Could you check a few things on this drawing? It's one solid part, dimensions in mm from its lowest x, y, z. A direction names the side the tool comes from. Round coordinates to 2 decimals unless told otherwise and drop trailing zeros. Loops run counter-clockwise (first coordinate to the right, second up) from the corner with the lowest first, then second, coordinate; pieces in that order, holes last. Notation, with made-up numbers: (50.5, -28.5) -> (99.5, -28.5) arc R21 cw to (99.5, 9.5) -> close; hole circle Ø6 at (-36, -6.5). An arc over 180 degrees is marked (long way). Use CSV: the item, a comma, the result in double quotes. Start each with the question number.
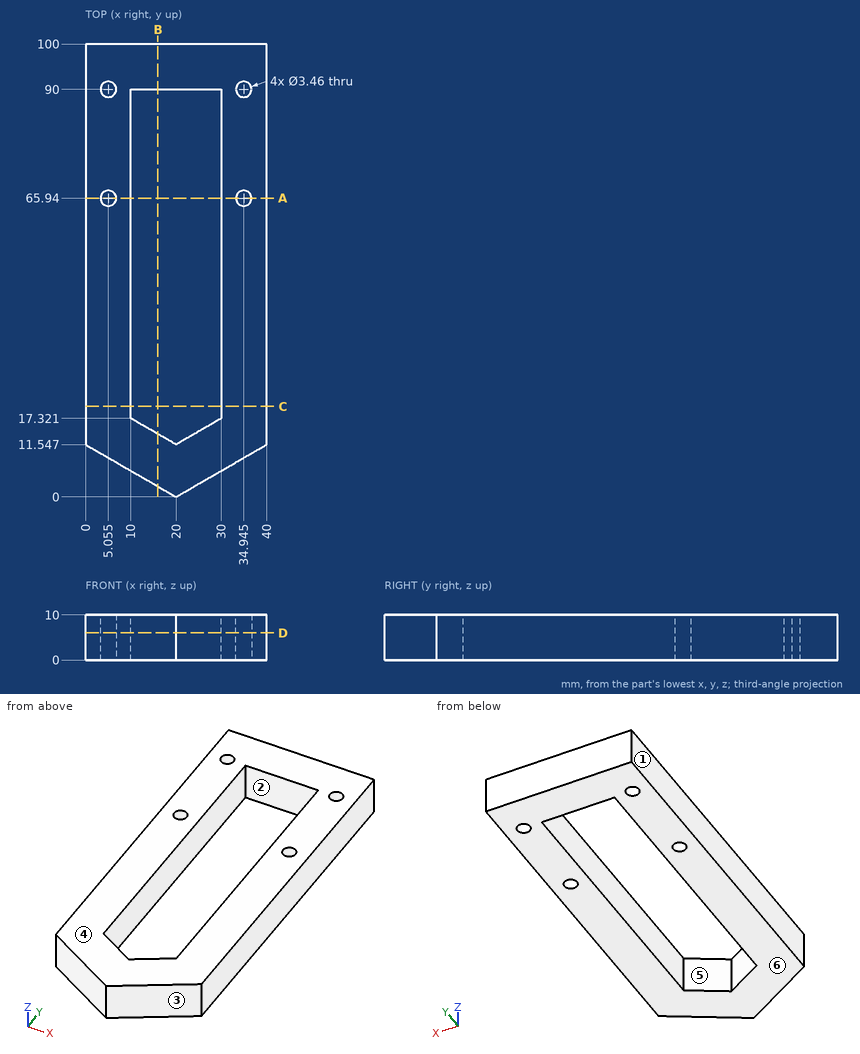
Q1. I need wall thicknesses on line 1 along Y through (x, z) = (20, 9) (1 decimal); line 2 along X through (y, z) = (54, 5.5); line 3 along X through (y, z) = (90.5, 4.25). Which ranges of each line are inside material? Lowest first, please.
Q2. I want a section at A-A, the plane y = 65.94. List the corners of the cut face in (x, z) for me (1 decimal).
Q3. I want a section at C-C, the plane y = 20. List the corners of the cut face in (x, z) for me.
Q4. I want a section at D-D, the plane z = 6. List the corners of the cut face in (x, y) for me (1 decimal).
Q5. For the marked faces 5 and 6, which set-ups out of +Z, -Z, +X, -X, +Y, -Y let a thin tool reach every point of the face, with its end or its side?
Q6. Will this pin go through, and if not, where does the flat tip stop? pin 1 Ø2 at (x, z) = (12.5, 7) entering from -Y.
Q7. If we mould it in two halves opening along X, with no side actions, what happens to the marked faces 1, 2, 3 and 4? For each: pulls with the +X half, pulls with the -X half, needs draft (parallel to the pull), parting line crosses it, or undercut.
Q8. I want a section at B-B, the plane x = 16. List the corners of the cut face in (y, z) for me.
Values found:
1,line 1,"0 to 11.5, 90 to 100"
1,line 2,"0 to 10, 30 to 40"
1,line 3,"0 to 3.4, 6.71 to 33.29, 36.6 to 40"
2,outline,"(0, 0) -> (3.3, 0) -> (3.3, 10) -> (0, 10) -> close; (6.8, 0) -> (10, 0) -> (10, 10) -> (6.8, 10) -> close; (30, 0) -> (33.2, 0) -> (33.2, 10) -> (30, 10) -> close; (36.7, 0) -> (40, 0) -> (40, 10) -> (36.7, 10) -> close"
3,outline,"(0, 0) -> (10, 0) -> (10, 10) -> (0, 10) -> close; (30, 0) -> (40, 0) -> (40, 10) -> (30, 10) -> close"
4,outline,"(0, 11.5) -> (20, 0) -> (40, 11.5) -> (40, 100) -> (0, 100) -> close; hole circle Ø3.5 at (5.1, 65.9); hole circle Ø3.5 at (5.1, 90); hole (10, 17.3) -> (20, 11.5) -> (30, 17.3) -> (30, 90) -> (10, 90) -> close; hole circle Ø3.5 at (34.9, 65.9); hole circle Ø3.5 at (34.9, 90)"
5,face 5,"+Z, -Z"
5,face 6,"-Z, +X, -X, +Y, -Y"
6,pin 1,"y = 3.75"
7,face 1,"pulls with the -X half"
7,face 2,"undercut"
7,face 3,"pulls with the +X half"
7,face 4,"needs draft"
8,outline,"(2.31, 0) -> (13.86, 0) -> (13.86, 10) -> (2.31, 10) -> close; (90, 0) -> (100, 0) -> (100, 10) -> (90, 10) -> close"
